Work out the finished part from the listing and answer in its coordinate system (mm). Give positions to 0.01 mm unless a question says otherwise; leave off trailing zeros. Loops run counter-clockwise (first coordinate to the right, second up) from the corner with the lowest first, then second, coordinate; pieces in that order, holes last. Notation, with made-up numbers: M 21,63 L 55,63 A20 ccw 55,102 Z; hole C 47,26 d7. An arc over 180 degrees is marked long. Answer in a Markdown table with one row per item. Add a question column.
from build123d import *

# Parameters (mm, degrees)
BOSS_EXTRUDE1_DEPTH = 1.905
CUT_EXTRUDE1_DEPTH  = 36.971502957


with BuildPart() as part:
    # Sketch1 → Boss-Extrude1 (new body)
    with BuildSketch(Plane(origin=(0, 0, 0), x_dir=(1, 0, 0), z_dir=(0, 1, 0))):
        with BuildLine():
            Line((0.635, 0), (24.765, 0))
            ThreePointArc((24.765, 0), (25.214012806, 0.185987194), (25.4, 0.635))
            Line((25.4, 0.635), (25.4, 24.765))
            ThreePointArc((25.4, 24.765), (25.214012806, 25.214012806), (24.765, 25.4))
            Line((24.765, 25.4), (0.635, 25.4))
            ThreePointArc((0.635, 25.4), (0.185987194, 25.214012806), (0, 24.765))
            Line((0, 24.765), (0, 0.635))
            ThreePointArc((0, 0.635), (0.185987194, 0.185987194), (0.635, 0))
        make_face()
    extrude(amount=BOSS_EXTRUDE1_DEPTH)

    # Sketch2 → Cut-Extrude1 (cut, through all)
    with BuildSketch(Plane(origin=(0, 1.905, 0), x_dir=(1, 0, 0), z_dir=(0, 1, 0))):
        with BuildLine():
            Line((10.1346, 2.8194), (15.2654, 2.8194))
            ThreePointArc((15.2654, 2.8194), (15.355202561, 2.856597439), (15.3924, 2.9464))
            Line((15.3924, 2.9464), (15.3924, 5.6642))
            ThreePointArc((15.3924, 5.6642), (14.648451224, 7.460251224), (12.8524, 8.2042))
            Line((12.8524, 8.2042), (12.5476, 8.2042))
            ThreePointArc((12.5476, 8.2042), (10.751548776, 7.460251224), (10.0076, 5.6642))
            Line((10.0076, 5.6642), (10.0076, 2.9464))
            ThreePointArc((10.0076, 2.9464), (10.044797439, 2.856597439), (10.1346, 2.8194))
        make_face()
        with BuildLine():
            Line((5.461, 20.955), (7.239, 20.955))
            ThreePointArc((7.239, 20.955), (7.328802561, 20.917802561), (7.366, 20.828))
            Line((7.366, 20.828), (7.366, 13.97))
            ThreePointArc((7.366, 13.97), (7.328802561, 13.880197439), (7.239, 13.843))
            Line((7.239, 13.843), (5.461, 13.843))
            ThreePointArc((5.461, 13.843), (5.371197439, 13.880197439), (5.334, 13.97))
            Line((5.334, 13.97), (5.334, 14.2875))
            Line((5.334, 14.2875), (3.3528, 14.2875))
            ThreePointArc((3.3528, 14.2875), (3.173194878, 14.361894878), (3.0988, 14.5415))
            Line((3.0988, 14.5415), (3.0988, 16.4465))
            ThreePointArc((3.0988, 16.4465), (3.173194878, 16.626105122), (3.3528, 16.7005))
            Line((3.3528, 16.7005), (5.334, 16.7005))
            Line((5.334, 16.7005), (5.334, 18.0975))
            Line((5.334, 18.0975), (3.3528, 18.0975))
            ThreePointArc((3.3528, 18.0975), (3.173194878, 18.171894878), (3.0988, 18.3515))
            Line((3.0988, 18.3515), (3.0988, 20.2565))
            ThreePointArc((3.0988, 20.2565), (3.173194878, 20.436105122), (3.3528, 20.5105))
            Line((3.3528, 20.5105), (5.334, 20.5105))
            Line((5.334, 20.5105), (5.334, 20.828))
            ThreePointArc((5.334, 20.828), (5.371197439, 20.917802561), (5.461, 20.955))
        make_face()
        with BuildLine():
            Line((18.161, 21.844), (19.939, 21.844))
            ThreePointArc((19.939, 21.844), (20.028802561, 21.806802561), (20.066, 21.717))
            Line((20.066, 21.717), (20.066, 20.5105))
            Line((20.066, 20.5105), (22.0472, 20.5105))
            ThreePointArc((22.0472, 20.5105), (22.226805122, 20.436105122), (22.3012, 20.2565))
            Line((22.3012, 20.2565), (22.3012, 18.3515))
            ThreePointArc((22.3012, 18.3515), (22.226805122, 18.171894878), (22.0472, 18.0975))
            Line((22.0472, 18.0975), (20.066, 18.0975))
            Line((20.066, 18.0975), (20.066, 16.7005))
            Line((20.066, 16.7005), (22.0472, 16.7005))
            ThreePointArc((22.0472, 16.7005), (22.226805122, 16.626105122), (22.3012, 16.4465))
            Line((22.3012, 16.4465), (22.3012, 14.5415))
            ThreePointArc((22.3012, 14.5415), (22.226805122, 14.361894878), (22.0472, 14.2875))
            Line((22.0472, 14.2875), (20.066, 14.2875))
            Line((20.066, 14.2875), (20.066, 13.081))
            ThreePointArc((20.066, 13.081), (20.028802561, 12.991197439), (19.939, 12.954))
            Line((19.939, 12.954), (18.161, 12.954))
            ThreePointArc((18.161, 12.954), (18.071197439, 12.991197439), (18.034, 13.081))
            Line((18.034, 13.081), (18.034, 21.717))
            ThreePointArc((18.034, 21.717), (18.071197439, 21.806802561), (18.161, 21.844))
        make_face()
    extrude(amount=-CUT_EXTRUDE1_DEPTH, mode=Mode.SUBTRACT)


solid = part.part
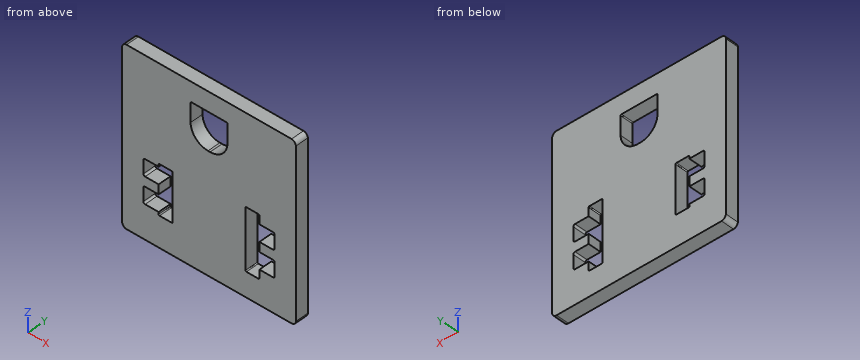
(1) Section B-B, the plane x = 6.5 is taken. Determine the outline of the cut face in (y, z) (3 decimals).
(2) Section D-D, the plane x = 21 is taken. Determine the outline of the cut face in (y, z) (1 decimal).
(3) Section C-C, the plane z = -15.25 is taken. Determine the outline of the cut face in (x, y) (3 decimals).
(4) Consider line 1 along X through (y, z) = (0.7, -14); line 2 along X through (y, z) = (1.75, -19.5); line 3 along Z through (x, y) = (5.75, 1.25) (3 decimals). Determine where each line is inside the solid, lowest interval first. Write a range as from..to.
(5) Section A-A, the plane z = -4.25 is taken. Determine the outline of the cut face in (x, y) (3 decimals).
Numbers:
| question | item | result |
|---|---|---|
| 1 | outline | M 0,-25.4 L 1.905,-25.4 L 1.905,-20.955 L 0,-20.955 Z; M 0,-13.843 L 1.905,-13.843 L 1.905,0 L 0,0 Z |
| 2 | outline | M 0,-25.4 L 1.9,-25.4 L 1.9,-20.5 L 0,-20.5 Z; M 0,-18.1 L 1.9,-18.1 L 1.9,-16.7 L 0,-16.7 Z; M 0,-14.3 L 1.9,-14.3 L 1.9,0 L 0,0 Z |
| 3 | outline | M 0,0 L 3.099,0 L 3.099,1.905 L 0,1.905 Z; M 7.366,0 L 18.034,0 L 18.034,1.905 L 7.366,1.905 Z; M 22.301,0 L 25.4,0 L 25.4,1.905 L 22.301,1.905 Z |
| 4 | line 1 | x = 0..5.33, 7.37..18.03, 20.07..25.4 |
| 4 | line 2 | x = 0..3.1, 7.37..18.03, 22.3..25.4 |
| 4 | line 3 | z = -25.4..-20.955, -13.843..0 |
| 5 | outline | M 0,0 L 10.008,0 L 10.008,1.905 L 0,1.905 Z; M 15.392,0 L 25.4,0 L 25.4,1.905 L 15.392,1.905 Z |
